```python
from build123d import *

# Parameters (mm, degrees)
F1_DEPTH = 38.1
F2_W     = 3.020811
F2_H     = 44.635244
F2_W_2   = 3.2222
F2_H_2   = 44.836629
F2_W_3   = 2.618038
F2_W_4   = 2.819423
F3_DEPTH = 5.08


with BuildPart() as f1:
    # F0 (on Front) → F1 (new body)
    with BuildSketch(Plane.XZ):
        Polygon((16.942143, 44.659857), (-36.352359, 44.659857), (-36.762383, -65.636605), (-17.255633, -97.091005), (-1.502697, -97.091005), (16.942143, -65.636605), align=None)
        with BuildLine():
            ThreePointArc((16.942143, 44.659857), (-9.705108, 62.248629), (-36.352359, 44.659857))
            Line((-36.352359, 44.659857), (16.942143, 44.659857))
        make_face()
        Polygon((-1.502697, -97.091005), (-17.255633, -97.091005), (-9.158776, -110.147089), align=None)
    extrude(amount=F1_DEPTH)

    # F2 (on face) → F3 (join)
    with BuildSketch(Plane.XZ.offset(38.1)):
        Polygon((-24.548945, 44.838252), (-28.140236, 44.635244), (-28.306166, 0), (-24.71568, -0.013348), align=None)
        with Locations((-19.581269, 22.317622)):
            Rectangle(F2_W, F2_H)
        with Locations((-13.036178, 22.418314)):
            Rectangle(F2_W_2, F2_H_2)
        with Locations((-6.491086, 22.418314)):
            Rectangle(F2_W_3, F2_H_2)
        with Locations((4.887302, 22.418314)):
            Rectangle(F2_W_4, F2_H_2)
    extrude(amount=F3_DEPTH)


solid = f1.part
```
For this review, take the finished solid that the model builds, in its own axes (mm). A direction names the side the tool comes from. Coordinates: 2 decimals unless noted, no trailing zeros. Order: outer loops, then holes, each group sorted by start corner. A loop starts at its lowest first (then second) coordinate and runs counter-clockwise, first axis right, second up. Notation, with made-up numbers: (-11, 24.5) -> (38, 24.5) arc R17 ccw to (38, 43.5) -> close; hole circle Ø9 at (28, 36.25). An arc over 180 degrees is marked (long way). Answer as CSV lines item,"result".
Q1. Wall thickness on line 1 along Y through (x, z) = (-10.5, 8.5); line 2 along X through (y, z) = (-19, 33); line 3 along X through (y, z) = (-12.5, 45.5): over which ranges is each line inside the solid? List them lowest first. Write a range as [from, to].
Model answer:
line 1,"y = [-38.1, 0]"
line 2,"x = [-36.4, 16.94]"
line 3,"x = [-35.98, 16.57]"
Q2. Clearance check with flat-ended pins moving along their axes: pin 1 Ø2 at (x, y) = (-6, -41.5) entering from +Z; pin 2 Ø8 at (x, z) = (3, -89) entering from +Y; pin 3 Ø4 at (y, z) = (-40, 12.5) entering from -X; pin 4 Ø2.5 at (y, z) = (-40, 23.5) entering from -X. State where each tip first meets the part, or that it passes through.
Model answer:
pin 1,"stops at z = 44.84"
pin 2,"stops at y = 0"
pin 3,"stops at x = -36.47"
pin 4,"stops at x = -28.22"
Q3. We need section C-C (x = 10.5). State the section outline as (y, z) points.
Model answer:
outline,"(-38.1, -76.62) -> (0, -76.62) -> (0, 54.04) -> (-38.1, 54.04) -> close"
Q4. We need section A-A (y = -15). State the section outline as (x, z) points.
Model answer:
outline,"(-36.76, -65.64) -> (-9.16, -110.15) -> (16.94, -65.64) -> (16.94, 44.66) arc R28.98 ccw to (-36.35, 44.66) -> close"
Q5. For faces 1 (the face through (-13, -41, 0)), 2 (the face through (-13, -43.18, 23)), 3 (the face through (-13, -41, 44.837)), 4 (the face through (3.478, -41, 22)), list the 3-axis set-ups (+Z, -Z, +X, -X, +Y, -Y) from which the entire face can be reached by the end or side of a thin tool; tool diameter is ignored.
Model answer:
face 1,"-Z, +X, -X, -Y"
face 2,"+Z, -Z, +X, -X, -Y"
face 3,"+Z, +X, -X, -Y"
face 4,"+Z, -Z, -Y"
Q6. Draft analysis for pull direction X (two halves, no side actions). For faces 5 (the face through (-20, -41, 44.635)), 6 (the face through (-20, -41, 0)), 7 (the face through (-26.32, -40.6, 44.74)), state which applies: released by +X, released by -X, zero draft, split by the parting line, or undercut.
Model answer:
face 5,"undercut"
face 6,"zero draft"
face 7,"released by -X"
Q7. We need section D-D (z = -63.5). State the section outline as (x, y) points.
Model answer:
outline,"(-36.75, -38.1) -> (16.94, -38.1) -> (16.94, 0) -> (-36.75, 0) -> close"
Q8. We need section B-B (z = 19.5). State the section outline as (x, y) points.
Model answer:
outline,"(-36.45, -38.1) -> (-28.23, -38.1) -> (-28.23, -43.18) -> (-24.64, -43.18) -> (-24.64, -38.1) -> (-21.09, -38.1) -> (-21.09, -43.18) -> (-18.07, -43.18) -> (-18.07, -38.1) -> (-14.65, -38.1) -> (-14.65, -43.18) -> (-11.43, -43.18) -> (-11.43, -38.1) -> (-7.8, -38.1) -> (-7.8, -43.18) -> (-5.18, -43.18) -> (-5.18, -38.1) -> (3.48, -38.1) -> (3.48, -43.18) -> (6.3, -43.18) -> (6.3, -38.1) -> (16.94, -38.1) -> (16.94, 0) -> (-36.45, 0) -> close"
